Input: dimensioned drawing with shaded views. Units: mm. Origin: part minimum x, y, z. Round coordinates to 2 decimals unless told otherwise and drop trailing zeros. Loops run counter-clockwise (first coordinate to the right, second up) from the corner with the lowest first, then second, coordinate; pieces in that order, holes last. Notation, with made-up numbers: M 72.5,12 L 90.5,12 A9 ccw 90.5,25 Z; hole C -0.5,81 d6. An arc over 180 degrees is marked long. Answer as CSV lines item,"result". Start each with the question number.
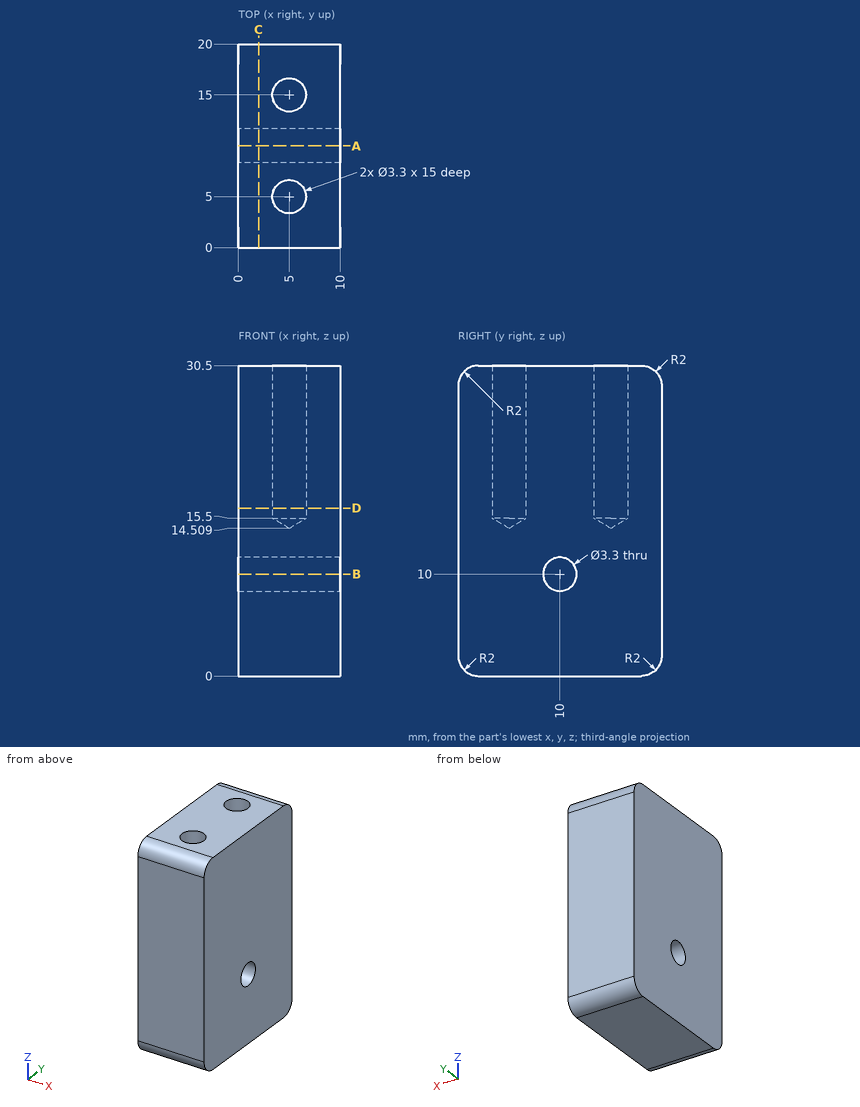
1) Section A-A, the plane y = 10. Return loops of the section in (x, z).
2) Contact query for flat-ended pins moving along their axis: pin 1 Ø1 at (y, z) = (11.5, 25) entering from -X; pin 2 Ø3 at (x, y) = (5, 5) entering from +Z. Output: stop coordinate, or through.
3) Section C-C, the plane x = 2. Return loops of the section in (y, z).
4) Ray query, line 1 along Y through (x, z) = (5, 16); line 2 along Y through (x, z) = (5.5, 10); line 3 along X through (y, z) = (5, 20.5). Return the intervals inside material, ascending.
5) Section B-B, the plane z = 10. Return loops of the section in (x, y), and give its area (3 significant figures).
6) Section D-D, the plane z = 16.5. Return loops of the section in (x, y).
Findings below:
1,outline,"M 0,0 L 10,0 L 10,8.35 L 0,8.35 Z; M 0,11.65 L 10,11.65 L 10,30.5 L 0,30.5 Z"
2,pin 1,"x = 0"
2,pin 2,"z = 15.41"
3,outline,"M 0,2 A2 ccw 2,0 L 18,0 A2 ccw 20,2 L 20,28.5 A2 ccw 18,30.5 L 2,30.5 A2 ccw 0,28.5 Z; hole C 10,10 d3.3"
4,line 1,"0 to 3.35, 6.65 to 13.35, 16.65 to 20"
4,line 2,"0 to 8.35, 11.65 to 20"
4,line 3,"0 to 3.35, 6.65 to 10"
5,outline,"M 0,0 L 10,0 L 10,8.35 L 0,8.35 Z; M 0,11.65 L 10,11.65 L 10,20 L 0,20 Z"
5,area,"167 mm²"
6,outline,"M 0,0 L 10,0 L 10,20 L 0,20 Z; hole C 5,5 d3.3; hole C 5,15 d3.3"
